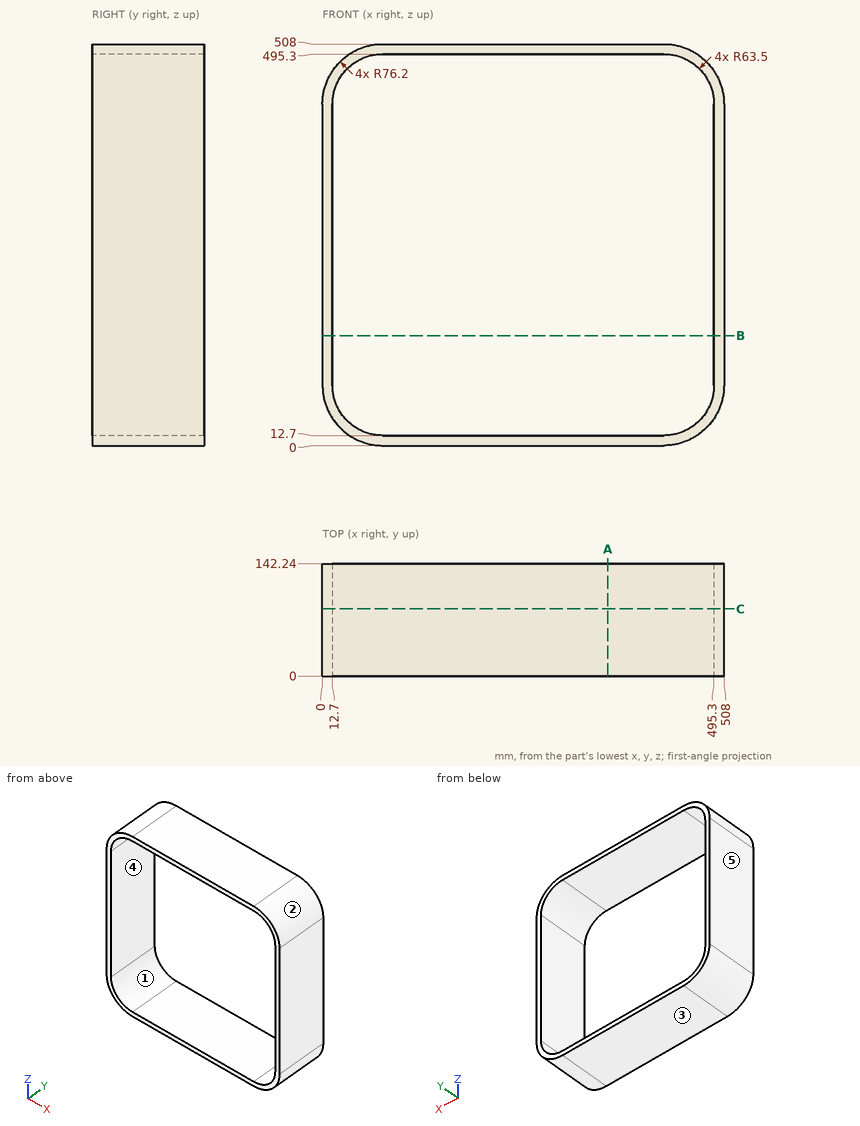
Geometry: see drawing. Coordinates: mm, zero at the bounding-box minimum. A direction names the side the tool comes from. Coordinates: 2 decimals unless noted, no trailing zeros. Loops run counter-clockwise (first coordinate to the right, second up) from the corner with the lowest first, then second, coordinate; pieces in that order, holes last. Notation, with made-up numbers: (14, 18.25) - (58, 18.25) arc R36 ccw to (58, 55.25) - close; hole circle Ø5 at (0.25, -27.5). An arc over 180 degrees is marked (long way). Answer in a Markdown table with one row per item.
(1) Cut plane A-A on x = 361. Output: boundary loops of the cut face in (y, z), plus the area to 3 significant figures.
Model answer:
| item | result |
|---|---|
| outline | (0, 0) - (142.24, 0) - (142.24, 12.7) - (0, 12.7) - close; (0, 495.3) - (142.24, 495.3) - (142.24, 508) - (0, 508) - close |
| area | 3,610 mm² |
(2) Cut plane C-C on y = 85. Output: boundary loops of the cut face in (x, z).
Model answer:
| item | result |
|---|---|
| outline | (0, 76.2) arc R76.2 ccw to (76.2, 0) - (431.8, 0) arc R76.2 ccw to (508, 76.2) - (508, 431.8) arc R76.2 ccw to (431.8, 508) - (76.2, 508) arc R76.2 ccw to (0, 431.8) - close; hole (12.7, 76.2) arc R63.5 ccw to (76.2, 12.7) - (431.8, 12.7) arc R63.5 ccw to (495.3, 76.2) - (495.3, 431.8) arc R63.5 ccw to (431.8, 495.3) - (76.2, 495.3) arc R63.5 ccw to (12.7, 431.8) - close |
(3) Pin query (flat end, axial travel): P1, Ø5, axis at x = 443.5, y = 24, coming from the +Z side; P2, Ø6, axis at x = 58.5, y = 124.5, coming from the +Z side. Return the tip coordinate at first contact, or that it passes through.
Model answer:
| item | result |
|---|---|
| P1 | stops at z = 507.44 |
| P2 | stops at z = 506.57 |
(4) Mould query, pull axis X, two halves, no side actions, for the marked faces 3, 4 and 5. Classes: pulls with the +X half, pulls with the -X half, needs draft (parallel to the pull), parting line crosses it, or undercut.
Model answer:
| item | result |
|---|---|
| face 3 | needs draft |
| face 4 | undercut |
| face 5 | pulls with the -X half |
(5) Material intervals for L1, parallel to Z at x = 154, y = 64; L2, parallel to X at y = 131.5, z = 26, sorted ascending. Write a range as from..to.
Model answer:
| item | result |
|---|---|
| L1 | z = 0..12.7, 495.3..508 |
| L2 | x = 18.87..37.31, 470.69..489.13 |
(6) Set-up query: the marked faces 1 and 2. Return all of +Z, -Z, +X, -X, +Y, -Y with unobstructed straight access to the full face (end or side cutting, diameter ignored); none if empty.
Model answer:
| item | result |
|---|---|
| face 1 | +Y, -Y |
| face 2 | +Z, +X, +Y, -Y |
(7) Cut plane B-B on z = 139. Output: boundary loops of the cut face in (x, y).
Model answer:
| item | result |
|---|---|
| outline | (0, 0) - (12.7, 0) - (12.7, 142.24) - (0, 142.24) - close; (495.3, 0) - (508, 0) - (508, 142.24) - (495.3, 142.24) - close |
